Source: three-view drawing plus pictorial views. Frame: mm from the lowest corner of the part. A direction names the side the tool comes from. Give positions to 0.01 mm unless a question says otherwise; leave off trailing zeros. Order: outer loops, then holes, each group sorted by start corner. A loop starts at its lowest first (then second) coordinate and runs counter-clockwise, first axis right, second up.
1) Material intervals for line 1 (X direction, y = 4, z = 4); line 2 (X direction, y = 5, z = 27.65); line 3 (Z direction, x = 26.5, y = 7.75), sorted ascending.
2) Section A-A, the plane x = 27.5. Return loops of the section in (y, z).
3) Access query for the marked faces 1 and 2. Directions: +Z, -Z, +X, -X, +Y, -Y. A direction counts if a zero-diameter tool reaches every point of the face in a straight line with its end or side. Return the directions, or none.
4) First-contact query: P1, Ø2, axis at x = 27.5, z = 27.5, coming from the +Y side. Flat tip, straight axial feed; report the tip coordinate or a pass-through.
5) Section C-C, the plane z = 28. Return loops of the section in (x, y).
6) Draft query along Z for the marked faces 3, 4 and 5. Return one class per face: released by +Z, released by -Z, zero draft, split by the parting line, or undercut.
7) Section B-B, the plane y = 1.75. Return loops of the section in (x, z).
8) Section D-D, the plane x = 15.75. Return loops of the section in (y, z), plus the area to 3 significant figures.
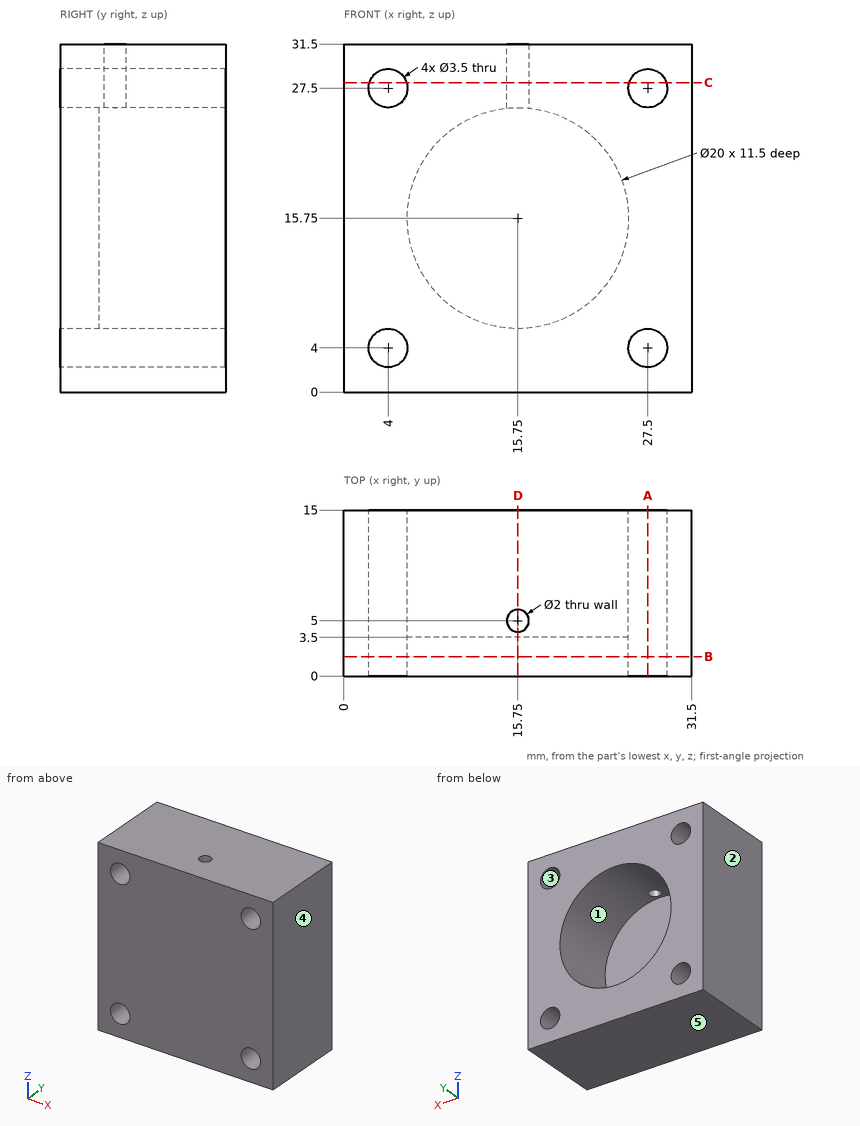
From the geometry:
1. line 1: x = 0 to 2.25, 5.75 to 25.75, 29.25 to 31.5
1. line 2: x = 0 to 2.26, 5.74 to 14.75, 16.75 to 25.76, 29.24 to 31.5
1. line 3: z = 0 to 2.56, 5.44 to 26.06, 28.94 to 31.5
2. outline: (0, 0) - (15, 0) - (15, 2.25) - (0, 2.25) - close; (0, 5.75) - (15, 5.75) - (15, 25.75) - (0, 25.75) - close; (0, 29.25) - (15, 29.25) - (15, 31.5) - (0, 31.5) - close
3. face 1: +Y
3. face 2: +Z, -Z, -X, +Y, -Y
4. P1: passes through
5. outline: (0, 0) - (2.32, 0) - (2.32, 15) - (0, 15) - close; (5.68, 0) - (25.82, 0) - (25.82, 15) - (5.68, 15) - close; (29.18, 0) - (31.5, 0) - (31.5, 15) - (29.18, 15) - close; hole circle Ø2 at (15.75, 5)
6. face 3: undercut
6. face 4: zero draft
6. face 5: released by -Z
7. outline: (0, 0) - (31.5, 0) - (31.5, 31.5) - (0, 31.5) - close; hole circle Ø3.5 at (4, 4); hole circle Ø3.5 at (4, 27.5); hole circle Ø3.5 at (27.5, 4); hole circle Ø3.5 at (27.5, 27.5)
8. outline: (0, 0) - (15, 0) - (15, 5.75) - (3.5, 5.75) - (3.5, 25.75) - (4, 25.75) - (4, 31.5) - (0, 31.5) - close; (6, 25.75) - (15, 25.75) - (15, 31.5) - (6, 31.5) - close
8. area: 231 mm2
